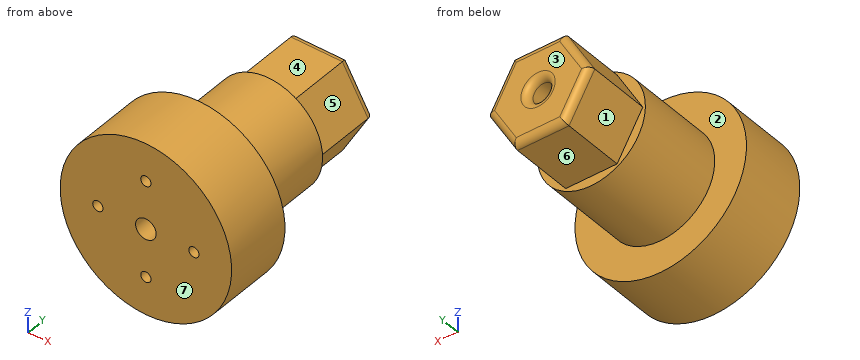
```python
from build123d import *

# Parameters (mm, degrees)
CROQUIS1_R              = 12.5
CROQUIS1_R_2            = 0.75
SALIENTE_EXTRUIR1_DEPTH = 10
CROQUIS2_R              = 7.875
SALIENTE_EXTRUIR2_DEPTH = 13
SALIENTE_EXTRUIR3_DEPTH = 10
CROQUIS4_R              = 1.5
CORTAR_EXTRUIR1_DEPTH   = 38.436613095
REDONDEO1_R             = 1


with BuildPart() as part:
    # Croquis1 → Saliente-Extruir1 (new body)
    with BuildSketch(Plane(origin=(0, 0, 0), x_dir=(1, 0, 0), z_dir=(0, 1, 0))):
        with Locations(Location((0, 0, 0), (0, 0, 270))):
            Circle(CROQUIS1_R)
        with Locations(Location((7, 0, 0), (0, 0, 270))):
            Circle(CROQUIS1_R_2, mode=Mode.SUBTRACT)
        with Locations(Location((0, -7, 0), (0, 0, 270))):
            Circle(CROQUIS1_R_2, mode=Mode.SUBTRACT)
        with Locations(Location((-7, 0, 0), (0, 0, 270))):
            Circle(CROQUIS1_R_2, mode=Mode.SUBTRACT)
        with Locations(Location((0, 7, 0), (0, 0, 270))):
            Circle(CROQUIS1_R_2, mode=Mode.SUBTRACT)
    extrude(amount=SALIENTE_EXTRUIR1_DEPTH)

    # Croquis2 → Saliente-Extruir2 (add)
    with BuildSketch(Plane(origin=(0, 10, 0), x_dir=(1, 0, 0), z_dir=(0, 1, 0))):
        with Locations(Location((0, 0, 0), (0, 0, 90))):
            Circle(CROQUIS2_R)
    extrude(amount=SALIENTE_EXTRUIR2_DEPTH)

    # Croquis3 → Saliente-Extruir3 (add)
    with BuildSketch(Plane(origin=(0, 23, 0), x_dir=(1, 0, 0), z_dir=(0, 1, 0))):
        Polygon((7.5, 0), (3.75, 6.495190528), (-3.75, 6.495190528), (-7.5, 0), (-3.75, -6.495190528), (3.75, -6.495190528), align=None)
    extrude(amount=SALIENTE_EXTRUIR3_DEPTH)

    # Croquis4 → Cortar-Extruir1 (cut, through all)
    with BuildSketch(Plane(origin=(0, 33, 0), x_dir=(1, 0, 0), z_dir=(0, 1, 0))):
        with Locations(Location((0, 0, 0), (0, 0, 270))):
            Circle(CROQUIS4_R)
    extrude(amount=-CORTAR_EXTRUIR1_DEPTH, mode=Mode.SUBTRACT)

    # Redondeo1
    redondeo1_edges = [part.edges().sort_by_distance(p)[0] for p in [
        (5.625, 33, 3.247595264),
        (5.625, 33, -3.247595264),
        (0, 33, -6.495190528),
        (-5.625, 33, -3.247595264),
        (-5.625, 33, 3.247595264),
        (0, 33, 6.495190528),
        (0, 33, -1.5),
    ]]
    fillet(redondeo1_edges, radius=REDONDEO1_R)


solid = part.part
```
The listing builds one solid part. Answer for the finished solid, in the listing's coordinates (mm). Face numbers are marked on the shaded views. A direction names the side the tool comes from. Round coordinates to 2 decimals unless told otherwise and drop trailing zeros. Write each loop counter-clockwise with the first axis right and the second up, starting at its lowest first coordinate (ties: lowest second). Pieces come first, ordered by that corner, then holes. Notation, with made-up numbers: (11.25, -5.5) -> (52.25, -5.5) arc R33 cw to (52.25, 33.5) -> close; hole circle Ø3 at (25.25, 2). An arc over 180 degrees is marked (long way). Use CSV: the item, a comma, the result in double quotes. Start each with the question number.
(1) Each of these flat-tipped pins is pushed along its axis until it touches: pin 1 (2.5 mm diameter, centred on x = 0, z = 0, fed in from -Y); pin 2 (0.9 mm diameter, centred on x = 0, z = 7, fed in from -Y); pin 3 (6 mm diameter, centred on y = 27, z = -6, fed in from +X); pin 4 (5 mm diameter, centred on x = 2, y = 17, fed in from -Z) (3 decimals). Where does it stop, or does it pass through?
(2) Section B-B on y = 26 is taken. Give the vertices of the cut face in (x, z).
(3) Section D-D on x = -10 is taken. Give the vertices of the cut face in (y, z).
(4) The mould has two halves that part along Z. Classify the marked faces 5, 6 and 7: released by +Z, released by -Z, zero draft, split by the parting line, or undercut.
(5) Consider L1, parallel to X at y = 7.5, z = 0; L2, parallel to X at y = 15.5, z = 0 (3 decimals); L3, parallel to Z at x = 10, y = 5.5. Determine where each line is inside the solid, lowest interval first. Write a range as from..to.
(6) Section C-C on z = -7 is taken. Give the vertices of the cut face in (x, y), then the cut area to 3 significant figures.
(7) Which of the six approach directions +Z, -Z, +X, -X, +Y, -Y give full straight-line access (tool end or side, diameter ignored) to the marked faces 1, 2, 3 and 4?
(8) Section A-A on x = 0 is taken. Give the vertices of the cut face in (y, z) (3 decimals), then the cut area to 3 significant figures.
A:
1,pin 1,"passes through"
1,pin 2,"stops at y = 10"
1,pin 3,"stops at x = 5.77"
1,pin 4,"stops at z = -7.875"
2,outline,"(-7.5, 0) -> (-3.75, -6.5) -> (3.75, -6.5) -> (7.5, 0) -> (3.75, 6.5) -> (-3.75, 6.5) -> close; hole circle Ø3 at (0, 0)"
3,outline,"(0, -7.5) -> (10, -7.5) -> (10, 7.5) -> (0, 7.5) -> close"
4,face 5,"released by +Z"
4,face 6,"released by -Z"
4,face 7,"zero draft"
5,L1,"x = -12.5..-7.75, -6.25..-1.5, 1.5..6.25, 7.75..12.5"
5,L2,"x = -7.875..-1.5, 1.5..7.875"
5,L3,"z = -7.5..7.5"
6,outline,"(-10.36, 0) -> (-0.75, 0) -> (-0.75, 10) -> (0.75, 10) -> (0.75, 0) -> (10.36, 0) -> (10.36, 10) -> (3.61, 10) -> (3.61, 23) -> (-3.61, 23) -> (-3.61, 10) -> (-10.36, 10) -> close"
6,area,"286 mm²"
7,face 1,"-Z, -X, +Y"
7,face 2,"+Y"
7,face 3,"+Z, -Z, +X, -X, +Y"
7,face 4,"+Z, +X, -X, +Y"
8,outline,"(0, -12.5) -> (10, -12.5) -> (10, -7.875) -> (23, -7.875) -> (23, -6.495) -> (32, -6.495) arc R1 ccw to (33, -5.495) -> (33, -2.5) arc R1 ccw to (32, -1.5) -> (0, -1.5) -> (0, -6.25) -> (10, -6.25) -> (10, -7.75) -> (0, -7.75) -> close; (0, 1.5) -> (32, 1.5) arc R1 ccw to (33, 2.5) -> (33, 5.495) arc R1 ccw to (32, 6.495) -> (23, 6.495) -> (23, 7.875) -> (10, 7.875) -> (10, 12.5) -> (0, 12.5) -> (0, 7.75) -> (10, 7.75) -> (10, 6.25) -> (0, 6.25) -> close"
8,area,"455 mm²"
